from build123d import *

# Parameters (mm, degrees)
F0_W      = 30
F0_H      = 40
F1_DEPTH  = 10
F2_W      = 20
F2_H      = 40
F3_DEPTH  = 0.5
F4_W      = 6.5
F4_H      = 10
F5_DEPTH  = 3
F6_W      = 6.5
F6_H      = 10
F7_DEPTH  = 3
F8_W      = 20
F8_H      = 10
F9_DEPTH  = 15
F11_D     = 5.5
F13_D     = 9
F13_DEPTH = 5
F13_TIP   = 2.7038727856
F15_D     = 11
F15_DEPTH = 3
F15_TIP   = 3.3047334047
F17_D     = 11
F17_DEPTH = 3
F17_TIP   = 3.3047334047
F19_D     = 3.3
F19_DEPTH = 30
F19_TIP   = 0.9914200214
F21_D     = 6
F21_DEPTH = 3
F21_TIP   = 1.8025818571


with BuildPart() as f1:
    # F0 (on Front) → F1 (new body)
    with BuildSketch(Plane.XZ):
        Rectangle(F0_W, F0_H)
    extrude(amount=F1_DEPTH)

    # F2 (on face) → F3 (cut)
    with BuildSketch(Plane(origin=(0, 0, 0), x_dir=(-1, 0, 0), z_dir=(0, 1, 0))):
        Rectangle(F2_W, F2_H)
    extrude(amount=-F3_DEPTH, mode=Mode.SUBTRACT)

    # F4 (on face) → F5 (cut)
    with BuildSketch(Plane(origin=(0, -0.5, 0), x_dir=(-1, 0, 0), z_dir=(0, 1, 0))):
        with Locations((-4.25, 15)):
            Rectangle(F4_W, F4_H)
    extrude(amount=-F5_DEPTH, mode=Mode.SUBTRACT)

    # F6 (on face) → F7 (cut)
    with BuildSketch(Plane(origin=(0, -0.5, 0), x_dir=(-1, 0, 0), z_dir=(0, 1, 0))):
        with Locations((-4.25, -15)):
            Rectangle(F6_W, F6_H)
    extrude(amount=-F7_DEPTH, mode=Mode.SUBTRACT)

    # F8 (on face) → F9 (join)
    with BuildSketch(Plane.XZ.offset(10)):
        with Locations((0, -15)):
            Rectangle(F8_W, F8_H)
    extrude(amount=F9_DEPTH)

    # F11 (through all)
    with Locations(Plane.XY.offset(-10)):
        with Locations((0, -17.5)):
            Hole(F11_D / 2)

    # F13
    with Locations(Plane.XY.offset(-10)):
        with Locations((0, -17.5)):
            Hole(F13_D / 2, depth=F13_DEPTH)
            with Locations((0, 0, -(F13_DEPTH + F13_TIP / 2))):  # 118° drill point
                Cone(0, F13_D / 2, F13_TIP, mode=Mode.SUBTRACT)

    # F15
    with Locations(Plane(origin=(0, -0.5, 0), x_dir=(-1, 0, 0), z_dir=(0, 1, 0))):
        with Locations((-4.25, 10)):
            Hole(F15_D / 2, depth=F15_DEPTH)
            with Locations((0, 0, -(F15_DEPTH + F15_TIP / 2))):  # 118° drill point
                Cone(0, F15_D / 2, F15_TIP, mode=Mode.SUBTRACT)

    # F17
    with Locations(Plane(origin=(0, -0.5, 0), x_dir=(-1, 0, 0), z_dir=(0, 1, 0))):
        with Locations((-4.25, -10)):
            Hole(F17_D / 2, depth=F17_DEPTH)
            with Locations((0, 0, -(F17_DEPTH + F17_TIP / 2))):  # 118° drill point
                Cone(0, F17_D / 2, F17_TIP, mode=Mode.SUBTRACT)

    # F19
    with Locations(Plane(origin=(0, -0.5, 0), x_dir=(-1, 0, 0), z_dir=(0, 1, 0))):
        with Locations((0, 0)):
            Hole(F19_D / 2, depth=F19_DEPTH)
            with Locations((0, 0, -(F19_DEPTH + F19_TIP / 2))):  # 118° drill point
                Cone(0, F19_D / 2, F19_TIP, mode=Mode.SUBTRACT)

    # F21
    with Locations(Plane.XZ.offset(10)):
        with Locations((0, 0)):
            Hole(F21_D / 2, depth=F21_DEPTH)
            with Locations((0, 0, -(F21_DEPTH + F21_TIP / 2))):  # 118° drill point
                Cone(0, F21_D / 2, F21_TIP, mode=Mode.SUBTRACT)


solid = f1.part
Model file for the job. Use its own axes, mm. A direction names the side the tool comes from. Give positions to 0.01 mm unless a question says otherwise; leave off trailing zeros. Order: outer loops, then holes, each group sorted by start corner. A loop starts at its lowest first (then second) coordinate and runs counter-clockwise, first axis right, second up. Notation, with made-up numbers: M 65.5,82 L 94.5,82 A11 cw 94.5,90 Z; hole C 5,76.25 d8. An arc over 180 degrees is marked long. Put each result on its own line as item: value. Start each with the question number.
(1) Pin check, flat tips, straight feed: pin 1 Ø1 at (x, z) = (6, -5.5) entering from +Y; pin 2 Ø6 at (x, y) = (-8.5, -18.5) entering from +Z; pin 3 Ø17.5 at (x, z) = (4.25, 10) entering from +Y; pin 4 Ø6 at (x, z) = (10.5, -2.5) entering from -Y. Stop position of each tip, or through.
(2) Band-saw the part on A-A on z = 0. Give the cut face in (x, y), then the cut area to 3 significant figures.
(3) Drill centre lines: L1, parallel to X at y = -17.5, z = -18.65; L2, parallel to Z at x = 0, y = -8.35; L3, parallel to X at y = -2, z = 18.5. Where is each one in solid material? Low to high. Write a range as [from, to].
(4) Tool access for faces 1 (the face through (1, -2, -17)), 2 (the face through (10, -17, -15)), 3 (the face through (4.443, -2.021, -4.503)), 4 (the face through (-2, -0.5, 0)): list every direction of +Z, -Z, +X, -X, +Y, -Y with a clear straight run to the whole face (end or side of a thin tool).
(5) Pull direction Y, two halves, no side cores. Call faces 5 (the face through (0.358, -14.773, -18.053)), 6 (the face through (0.59, -13.04, -12.54)), 7 (the face through (4, -3.5, 18)), 8 (the face through (1, -2, 17)): released by +Y, released by -Y, zero draft, split by the parting line, or undercut.
(6) Band-saw the part on D-D on x = 0. Count the separate pieces of the cut face and the enclosed holes in it, then the cut area to 3 significant figures.
(7) Band-saw the part on C-C on z = -4. Give the cut face in (x, y).
(8) Band-saw the part on B-B on y = -3. Give the cut face in (x, z), then the cut area to 3 significant figures.
Results below:
1. pin 1: stops at y = -3.6
1. pin 2: stops at z = -10
1. pin 3: stops at y = 0
1. pin 4: stops at y = -10
2. outline: M -15,-10 L -3,-10 L -3,-7 L -1.65,-6.19 L -1.65,-0.5 L -10,-0.5 L -10,0 L -15,0 Z; M 1.65,-6.19 L 3,-7 L 3,-10 L 15,-10 L 15,0 L 10,0 L 10,-0.5 L 1.65,-0.5 Z
2. area: 249 mm2
3. L1: x = [-10, -2.75], [2.75, 10]
3. L2: z = [-20, -3], [3, 20]
3. L3: x = [-15, 1], [7.5, 15]
4. face 1: -Z, +Y
4. face 2: +Z, -Z, +X, -Y
4. face 3: +Y
4. face 4: +Z, -Z, +Y
5. face 5: undercut
5. face 6: undercut
5. face 7: released by +Y
5. face 8: zero draft
6. separate pieces: 3
6. enclosed holes: 0
6. area: 366 mm2
7. outline: M -15,-10 L 15,-10 L 15,0 L 10,0 L 10,-0.5 L -10,-0.5 L -10,0 L -15,0 Z
8. outline: M -15,-20 L 1,-20 L 1,-14.44 A5.5 cw long 7.5,-14.44 L 7.5,-20 L 15,-20 L 15,20 L 7.5,20 L 7.5,14.44 A5.5 cw long 1,14.44 L 1,20 L -15,20 Z; hole C 0,0 d3.3
8. area: 938 mm2
